```python
from build123d import *

# Parameters (mm, degrees)
SKETCH1_W           = 38.4
SKETCH1_H           = 38.4
BOSS_EXTRUDE1_DEPTH = 6.5
FILLET1_R           = 3.5
SKETCH7_R           = 4
SKETCH7_R_2         = 2.75
CUT_EXTRUDE1_DEPTH  = 5.5
SKETCH8_R           = 2.75
CUT_EXTRUDE2_DEPTH  = 0.4


with BuildPart() as part:
    # Sketch1 → Boss-Extrude1 (new body)
    with BuildSketch(Plane(origin=(0, 0, 0), x_dir=(1, 0, 0), z_dir=(0, 1, 0))):
        with Locations((-19.2, -19.2)):
            Rectangle(SKETCH1_W, SKETCH1_H)
    extrude(amount=BOSS_EXTRUDE1_DEPTH)

    # Fillet1
    fillet1_edges = [part.edges().sort_by_distance(p)[0] for p in [
        (0, 3.25, 38.4),
        (-38.4, 3.25, 38.4),
        (-38.4, 3.25, 0),
        (0, 3.25, 0),
    ]]
    fillet(fillet1_edges, radius=FILLET1_R)

    # Sketch7 → Cut-Extrude1 (cut)
    with BuildSketch(Plane(origin=(0, 6.5, 0), x_dir=(1, 0, 0), z_dir=(0, 1, 0))):
        with BuildLine():
            Line((-3.5, -1.5), (-34.9, -1.5))
            ThreePointArc((-34.9, -1.5), (-36.314213562, -2.085786438), (-36.9, -3.5))
            Line((-36.9, -3.5), (-36.9, -34.9))
            ThreePointArc((-36.9, -34.9), (-36.314213562, -36.314213562), (-34.9, -36.9))
            Line((-34.9, -36.9), (-3.5, -36.9))
            ThreePointArc((-3.5, -36.9), (-2.085786438, -36.314213562), (-1.5, -34.9))
            Line((-1.5, -34.9), (-1.5, -3.5))
            ThreePointArc((-1.5, -3.5), (-2.085786438, -2.085786438), (-3.5, -1.5))
        make_face()
        with Locations((-19.2, -19.2)):
            Circle(SKETCH7_R, mode=Mode.SUBTRACT)
        with Locations((-29.7, -29.7)):
            Circle(SKETCH7_R, mode=Mode.SUBTRACT)
        with Locations((-8.7, -29.7)):
            Circle(SKETCH7_R, mode=Mode.SUBTRACT)
        with Locations((-8.7, -8.7)):
            Circle(SKETCH7_R, mode=Mode.SUBTRACT)
        with Locations((-29.7, -8.7)):
            Circle(SKETCH7_R, mode=Mode.SUBTRACT)
        with Locations((-29.7, -8.7)):
            Circle(SKETCH7_R_2)
        with Locations((-8.7, -8.7)):
            Circle(SKETCH7_R_2)
        with Locations((-19.2, -19.2)):
            Circle(SKETCH7_R_2)
        with Locations((-29.7, -29.7)):
            Circle(SKETCH7_R_2)
        with Locations((-8.7, -29.7)):
            Circle(SKETCH7_R_2)
    extrude(amount=-CUT_EXTRUDE1_DEPTH, mode=Mode.SUBTRACT)

    # Sketch8 → Cut-Extrude2 (cut)
    with BuildSketch(Plane(origin=(0, 1, 0), x_dir=(1, 0, 0), z_dir=(0, 1, 0))):
        with Locations((-29.7, -29.7)):
            Circle(SKETCH8_R)
        with Locations((-8.7, -29.7)):
            Circle(SKETCH8_R)
        with Locations((-8.7, -8.7)):
            Circle(SKETCH8_R)
        with Locations((-19.2, -19.2)):
            Circle(SKETCH8_R)
        with Locations((-29.7, -8.7)):
            Circle(SKETCH8_R)
    extrude(amount=-CUT_EXTRUDE2_DEPTH, mode=Mode.SUBTRACT)


solid = part.part
```
Input: part model. Units: mm. Frame: model coordinates. A direction names the side the tool comes from. Round coordinates to 2 decimals unless told otherwise and drop trailing zeros. Loops run counter-clockwise (first coordinate to the right, second up) from the corner with the lowest first, then second, coordinate; pieces in that order, holes last.
1) Pull-direction query (X, two-part tool) for faces 1 (the cylindrical face through (-12.696, 3.788, 8.524)), 2 (the flat face through (-19, 0, 19)), 3 (the cylindrical face through (-37.4, 3.3, 1.05)); classes: released by +X, released by -X, zero draft, split by the parting line, or undercut.
Ans:
face 1: undercut
face 2: zero draft
face 3: released by -X
2) Section query A-A on y = 4. Count the separate pieces of the cut face and the enclosed holes in it, plus the area to 3 significant figures.
Ans:
separate pieces: 6
enclosed holes: 6
area: 347 mm2
3) Section query C-C on z = 19.2. Return the cut outline in (x, y), plus the area to 4 significant figures.
Ans:
outline: (-38.4, 0) - (0, 0) - (0, 6.5) - (-1.5, 6.5) - (-1.5, 1) - (-15.2, 1) - (-15.2, 6.5) - (-16.45, 6.5) - (-16.45, 0.6) - (-21.95, 0.6) - (-21.95, 6.5) - (-23.2, 6.5) - (-23.2, 1) - (-36.9, 1) - (-36.9, 6.5) - (-38.4, 6.5) - close
area: 66.45 mm2
4) Section query B-B on x = -8.7. Return the cut outline in (y, z), plus the area to 3 significant figures.
Ans:
outline: (0, 0) - (6.5, 0) - (6.5, 1.5) - (1, 1.5) - (1, 4.7) - (6.5, 4.7) - (6.5, 5.95) - (0.6, 5.95) - (0.6, 11.45) - (6.5, 11.45) - (6.5, 12.7) - (1, 12.7) - (1, 25.7) - (6.5, 25.7) - (6.5, 26.95) - (0.6, 26.95) - (0.6, 32.45) - (6.5, 32.45) - (6.5, 33.7) - (1, 33.7) - (1, 36.9) - (6.5, 36.9) - (6.5, 38.4) - (0, 38.4) - close
area: 78.0 mm2
5) Set-up query: faces 4 (the cylindrical face through (-25.885, 3.788, 28.499)), 5 (the cylindrical face through (-37.4, 3.3, 37.35)). Return all of +Z, -Z, +X, -X, +Y, -Y with unobstructed straight access to the full face (end or side cutting, diameter ignored); none if empty.
Ans:
face 4: +Y
face 5: +Z, -X, +Y, -Y
6) Section query D-D on z = 8.7. Return the cut outline in (x, y).
Ans:
outline: (-38.4, 0) - (0, 0) - (0, 6.5) - (-1.5, 6.5) - (-1.5, 1) - (-4.7, 1) - (-4.7, 6.5) - (-5.95, 6.5) - (-5.95, 0.6) - (-11.45, 0.6) - (-11.45, 6.5) - (-12.7, 6.5) - (-12.7, 1) - (-25.7, 1) - (-25.7, 6.5) - (-26.95, 6.5) - (-26.95, 0.6) - (-32.45, 0.6) - (-32.45, 6.5) - (-33.7, 6.5) - (-33.7, 1) - (-36.9, 1) - (-36.9, 6.5) - (-38.4, 6.5) - close
7) Pin query (flat end, axial travel): pin 1 (4.5 mm diameter, centred on x = -8.7, z = 29.7, fed in from +Y); pin 2 (5 mm diameter, centred on x = -8.7, z = 8.7, fed in from -Y). Return the tip coordinate at first contact, or that it passes through.
Ans:
pin 1: stops at y = 0.6
pin 2: stops at y = 0
8) Material intervals for line 1 (Z direction, x = -8.7, y = 1.95); line 2 (X direction, y = 3.75, z = 19.2); line 3 (X direction, y = 3.55, z = 8.7), sorted ascending.
Ans:
line 1: z = 0 to 1.5, 4.7 to 5.95, 11.45 to 12.7, 25.7 to 26.95, 32.45 to 33.7, 36.9 to 38.4
line 2: x = -38.4 to -36.9, -23.2 to -21.95, -16.45 to -15.2, -1.5 to 0
line 3: x = -38.4 to -36.9, -33.7 to -32.45, -26.95 to -25.7, -12.7 to -11.45, -5.95 to -4.7, -1.5 to 0
